Answer from the drawing. Dimensions are ordinates in mm from the lowest x, y and z of the part. Round coordinates to 2 decimals unless told otherwise and drop trailing zeros. Write each loop counter-clockwise with the first axis right and the second up, starting at its lowest first coordinate (ties: lowest second). Pieces come first, ordered by that corner, then holes. Notation, with made-up numbers: (-14.5, 70) - (39.5, 70) arc R3 ccw to (39.5, 75) - close; hole circle Ø11 at (-6.75, 79). An arc over 180 degrees is marked (long way). Answer in a Markdown table with one row per item.
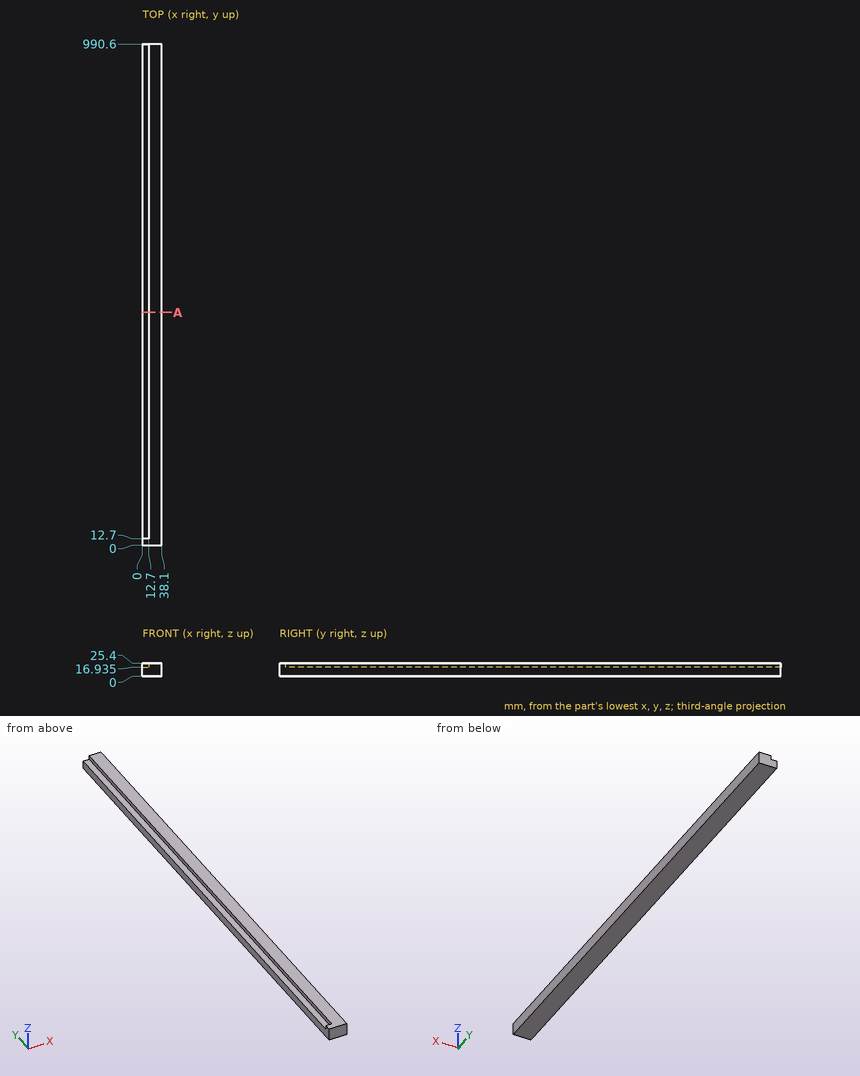
(1) Find the intervals of material crossed by line 1 (Z direction, x = 8, y = 639.5) (1 decimal); line 2 (Y direction, x = 7.5, z = 19.75); line 3 (X direction, y = 601, z = 21), in increasing order.
Checked values:
| item | result |
|---|---|
| line 1 | z = 0 to 16.9 |
| line 2 | y = 0 to 12.7 |
| line 3 | x = 12.7 to 38.1 |
(2) Flat-ended cylindrical pins translate along their axes: pin 1 (6 mm diameter, centred on x = 7, y = 122, fed in from +Z) (1 decimal); pin 2 (7 mm diameter, centred on y = 329, z = 21.5, fed in from -X); pin 3 (4 mm diameter, centred on x = 6.5, z = 21.5, fed in from +Y). Find the tip coordinate at first contact, or state that the pin passes through.
Checked values:
| item | result |
|---|---|
| pin 1 | stops at z = 16.9 |
| pin 2 | stops at x = 12.7 |
| pin 3 | stops at y = 12.7 |
(3) Section A-A (y = 460) is taken. Give the vertices of the cut face in (x, z) (1 decimal), and give its area (3 significant figures).
Checked values:
| item | result |
|---|---|
| outline | (0, 0) - (38.1, 0) - (38.1, 25.4) - (12.7, 25.4) - (12.7, 16.9) - (0, 16.9) - close |
| area | 860 mm2 |
